Here's how the part is built. I have some questions about the finished solid (model axes, mm). A direction names the side the tool comes from. Give positions to 0.01 mm unless a question says otherwise; leave off trailing zeros. Write each loop counter-clockwise with the first axis right and the second up, starting at its lowest first coordinate (ties: lowest second). Pieces come first, ordered by that corner, then holes. Notation, with made-up numbers: M 70,-12.75 L 120,-12.75 A19 cw 120,-2.75 Z; hole C 76.5,42.5 d3. An arc over 180 degrees is marked long. Answer as CSV lines item,"result". Start each with the question number.
Q1. For pin 1 (0.5 mm diameter, centred on y = -180.5, z = 0.5, fed in from -X); pin 2 (8 mm diameter, centred on x = 0.5, y = -187, fed in from -Z); pin 3 (0.5 mm diameter, centred on x = 1, z = 1, fed in from +Y), each with a flat end and sliding along its axis, tell me the tip position at first contact or that it passes through.
Q2. Suppose I cut it at C-C (z = 1.25). Write out the boundary of the cut face in (x, y).
Q3. If I drill on line 1 along Y through (x, z) = (-7.5, 1.4); line 2 along Y through (x, z) = (0.5, 0.4); line 3 along Y through (x, z) = (-0.5, 0.9), over which ranges is the centre line in solid material (lowest first)?
Q4. Thinking about a two-plate mould opening in Y: for faces 1 (the flat face through (-4, -184, 1.524)), 2 (the flat face through (1.524, -184, 1)), 3 (the cylindrical face through (-0.306, -216.096, 0.751)), which applies, +Y half, -Y half, draft (parallel to the pull), parting line (faces both ways), or undercut?
Q5. Suppose I cut it at B-B (x = -8.5). Write out the boundary of the cut face in (y, z).
Q6. On a 3-axis mill with a long thin cutter (end or side, diameter ignored), from which of +Z, -Z, +X, -X, +Y, -Y can I reach the whole of each face in a straight line? I mean faces 4 (the cylindrical face through (11.271, -160.326, 0.751)), 5 (the flat face through (0, -184, 1)). Say none if no direction works.
Q7. Suppose I cut it at D-D (x = 3). Write out the boundary of the cut face in (y, z).
Q8. Suppose I cut it at A-A (y = -159.5). Write out the boundary of the cut face in (x, z), then the cut area to 3 significant figures.
```python
from build123d import *

# Parameters (mm, degrees)
SKETCH1_W           = 1.524
SKETCH1_H           = 19.05
BOSS_EXTRUDE1_DEPTH = 1.524


with BuildPart() as part:
    # Sketch1 → Boss-Extrude1 (new body)
    with BuildSketch(Plane.XY):
        with BuildLine():
            Line((-11.16363506, -211.120891743), (-1.992949981, -216.780601905))
            ThreePointArc((-1.992949981, -216.780601905), (-0.281103266, -216.088759304), (1.524, -215.700600116))
            ThreePointArc((1.524, -215.700600116), (3.171388391, -214.980453866), (4.911266579, -214.527328034))
            ThreePointArc((4.911266579, -214.527328034), (8.56652215, -210.778134694), (8.366250568, -205.545808702))
            ThreePointArc((8.366250568, -205.545808702), (5.494506116, -190.54054727), (13.311403321, -177.414203341))
            ThreePointArc((13.311403321, -177.414203341), (14.109075531, -176.108897248), (14.468404268, -174.621958174))
            ThreePointArc((14.468404268, -174.621958174), (14.169609027, -170.480156419), (14.223154403, -166.327936138))
            ThreePointArc((14.223154403, -166.327936138), (14.204082667, -165.84665661), (14.094500503, -165.377630529))
            ThreePointArc((14.094500503, -165.377630529), (11.21769373, -160.262840376), (6.664633993, -156.56057856))
            ThreePointArc((6.664633993, -156.56057856), (2.313026504, -155.924450691), (-1.992949981, -155.030183999))
            ThreePointArc((-1.992949981, -155.030183999), (0.599102478, -159.944431448), (4.330540862, -164.060853624))
            ThreePointArc((4.330540862, -164.060853624), (-9.729681531, -161.306709082), (-21.139761832, -152.641535487))
            ThreePointArc((-21.139761832, -152.641535487), (-14.612667937, -165.552248896), (-2.254215141, -173.07276217))
            ThreePointArc((-2.254215141, -173.07276217), (-12.048739338, -189.17955679), (-5.548621032, -206.874471292))
            ThreePointArc((-5.548621032, -206.874471292), (-8.65863408, -208.597679765), (-11.16363506, -211.120891743))
        make_face()
        with Locations((0.762, -183.574694423)):
            Rectangle(SKETCH1_W, SKETCH1_H, mode=Mode.SUBTRACT)
    extrude(amount=BOSS_EXTRUDE1_DEPTH)


solid = part.part
```
Resolved:
1,pin 1,"x = -9.42"
1,pin 2,"z = 0"
1,pin 3,"y = -155.63"
2,outline,"M -21.14,-152.64 A26.36 ccw -2.25,-173.07 A21.71 ccw -5.55,-206.87 A12.6 ccw -11.16,-211.12 L -1.99,-216.78 A10.73 cw 1.52,-215.7 A11.44 cw 4.91,-214.53 A6.64 ccw 8.37,-205.55 A21.51 cw 13.31,-177.41 A4.93 ccw 14.47,-174.62 A48.92 cw 14.22,-166.33 A2.54 ccw 14.09,-165.38 A15.71 ccw 6.66,-156.56 A73.78 cw -1.99,-155.03 A22.19 ccw 4.33,-164.06 A31.69 cw Z; hole M 0,-193.1 L 1.52,-193.1 L 1.52,-174.05 L 0,-174.05 Z"
3,line 1,"-213.38 to -207.82, -204.71 to -177.86, -171 to -162.21"
3,line 2,"-215.88 to -193.1, -174.05 to -163.96, -159.8 to -155.58"
3,line 3,"-216.16 to -163.86, -158.21 to -155.37"
4,face 1,"draft"
4,face 2,"undercut"
4,face 3,"-Y half"
5,outline,"M -212.76,0 L -208.48,0 L -208.48,1.52 L -212.76,1.52 Z; M -203.33,0 L -179.24,0 L -179.24,1.52 L -203.33,1.52 Z; M -170.45,0 L -161.83,0 L -161.83,1.52 L -170.45,1.52 Z"
6,face 4,"+Z, -Z, +X, +Y"
6,face 5,"+Z, -Z"
7,outline,"M -215.04,0 L -164.08,0 L -164.08,1.52 L -215.04,1.52 Z; M -162.82,0 L -156.04,0 L -156.04,1.52 L -162.82,1.52 Z"
8,outline,"M -18.81,0 L -13.18,0 L -13.18,1.52 L -18.81,1.52 Z; M 0.3,0 L 10.53,0 L 10.53,1.52 L 0.3,1.52 Z"
8,area,"24.2 mm^2"
